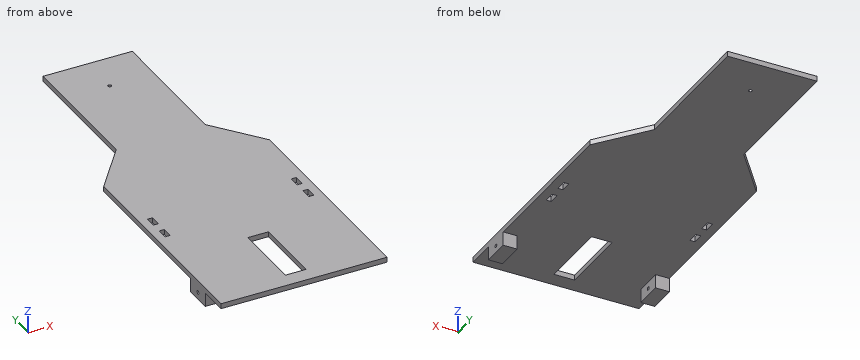
from build123d import *

# Parameters (mm, degrees)
F0_W     = 18.796
F0_H     = 40.64
F1_DEPTH = 18.796
F2_R     = 6.35
F3_DEPTH = 50.8
F4_W     = 101.6
F4_H     = 50.8
F4_R     = 6.35
F5_DEPTH = 50.8


# Not quite as in the source:
# - a feature names something its author has since deleted; it is built from what else it names


with BuildPart() as f1:
    # F0 (on Top) → F1 (new body)
    with BuildSketch(Plane.XY):
        Polygon((-163.8174757903, 706.2376797943), (-304.8, 526.2879983068), (-304.8, 30.9879983068), (-304.8, -286.5120016932), (304.8, -286.5120016932), (304.8, 30.9879983068), (304.8, 526.2879983068), (163.8174757903, 706.2376797943), (163.8174757903, 1214.2376797943), (-163.8174757903, 1214.2376797943), align=None)
        with Locations((-263.652, 180.8479983068)):
            Rectangle(F0_W, F0_H, mode=Mode.SUBTRACT)
        with Locations((-263.652, 262.1279983068)):
            Rectangle(F0_W, F0_H, mode=Mode.SUBTRACT)
        Polygon((38.1, 30.9879983068), (38.1, -229.3620016932), (-38.1, -229.3620016932), (-38.1, 30.9879983068), (0, 30.9879983068), align=None, mode=Mode.SUBTRACT)
        with Locations((263.652, 180.8479983068)):
            Rectangle(F0_W, F0_H, mode=Mode.SUBTRACT)
        with Locations((263.652, 262.1279983068)):
            Rectangle(F0_W, F0_H, mode=Mode.SUBTRACT)
        with BuildLine():
            ThreePointArc((0, 1055.4876797943), (-6.35, 1061.8376797943), (0, 1068.1876797943))
            ThreePointArc((0, 1068.1876797943), (4.4901280605, 1066.3278078548), (6.35, 1061.8376797943))
            ThreePointArc((6.35, 1061.8376797943), (4.4901280605, 1057.3475517337), (0, 1055.4876797943))
        make_face(mode=Mode.SUBTRACT)
    extrude(amount=F1_DEPTH)

    # F2 (on face) → F3 (join)
    with BuildSketch(Plane.YZ.offset(304.8)):
        Polygon((-127.7620016932, 0), (-178.5620016932, 0), (-178.5620016932, -50.8), (-127.7620016932, -50.8), (-76.9620016932, -50.8), (-76.9620016932, 0), align=None)
        with Locations((-127.7620016932, -25.4)):
            Circle(F2_R, mode=Mode.SUBTRACT)
    extrude(amount=-F3_DEPTH)

    # F4 (on face) → F5 (join)
    with BuildSketch(Plane(origin=(-304.8, 0, 0), x_dir=(0, -1, 0), z_dir=(-1, 0, 0))):
        with Locations((127.7626349211, -25.4)):
            Rectangle(F4_W, F4_H)
        with Locations((127.7626349211, -25.4)):
            Circle(F4_R, mode=Mode.SUBTRACT)
    extrude(amount=-F5_DEPTH)


solid = f1.part
Verification items for the finished model (mm, model axes). Round coordinates to 2 decimals unless told otherwise and drop trailing zeros. Write each loop counter-clockwise with the first axis right and the second up, starting at its lowest first coordinate (ties: lowest second). Pieces come first, ordered by that corner, then holes.
(1) Material ranges on line 1 (Y direction, x = -264, z = -25); line 2 (Y direction, x = 9, z = 6); line 3 (Z direction, x = 2, y = 900.5), recorded low to high.
Returned:
line 1: y = -178.56 to -134.1, -121.43 to -76.96
line 2: y = -286.51 to -229.36, 30.99 to 1214.24
line 3: z = 0 to 18.8
(2) Section check A-A (x = -110). Enter the section's corners in (y, z).
Returned:
outline: (-286.51, 0) - (1214.24, 0) - (1214.24, 18.8) - (-286.51, 18.8) - close
(3) Section check B-B (y = 834). Enter the section's corners in (x, z), plus the area to 3 significant figures.
Returned:
outline: (-163.82, 0) - (163.82, 0) - (163.82, 18.8) - (-163.82, 18.8) - close
area: 6,160 mm2
(4) Depth check by flat-ended pin: pin 1 Ø15 at (y, z) = (1039.5, 12) entering from -X; pin 2 Ø2 at (y, z) = (602, 1) entering from -X; pin 3 Ø15 at (x, z) = (283.5, -16.5) entering from +Y. Enter the tip coordinate at first touch or a pass-through.
Returned:
pin 1: stops at x = -163.82
pin 2: stops at x = -246.27
pin 3: stops at y = -76.96
